```python
from build123d import *

# Parameters (mm, degrees)
SCHIZZO1_R                    = 1.5
SCHIZZO1_W                    = 40
SCHIZZO1_H                    = 10
ESTRUSIONE_ESTRUSIONE1_DEPTH  = 4
RACCORDO1_R                   = 10
SCHIZZO2_R                    = 4
SCHIZZO2_R_2                  = 2
ESTRUSIONE_ESTRUSIONE2_DEPTH  = 4
SCHIZZO3_W                    = 40
SCHIZZO3_H                    = 5
ESTRUSIONE_ESTRUSIONE3_DEPTH  = 20
TAGLIO_ESTRUSIONE1_DEPTH      = 90.673017123
TAGLIO_ESTRUSIONE1_DEPTH_BACK = 90.673017123
SCHIZZO4_R                    = 2.5
SCHIZZO5_W                    = 5
SCHIZZO5_H                    = 60
ESTRUSIONE_ESTRUSIONE4_DEPTH  = 54
SCHIZZO6_R                    = 1.5
ESTRUSIONE_ESTRUSIONE5_DEPTH  = 5
RACCORDO2_R                   = 2
SMUSSO1_SIZE                  = 1
SCHIZZO7_R                    = 1
TAGLIO_ESTRUSIONE2_DEPTH      = 10


with BuildPart() as part:
    # Schizzo1 → Estrusione-Estrusione1 (new body)
    # profile 1 of 5: a face of its own
    with BuildSketch(Plane.XY):
        with BuildLine():
            Line((32.5, -20), (32.5, -10))
            Line((32.5, -10), (32.5, 10))
            Line((32.5, 10), (32.5, 20))
            Line((32.5, 20), (-64, 20))
            ThreePointArc((-64, 20), (-65.5, 18.5), (-67, 20))
            Line((-67, 20), (-72.5, 20))
            Line((-72.5, 20), (-72.5, -20))
            Line((-72.5, -20), (-67, -20))
            ThreePointArc((-67, -20), (-65.5, -18.5), (-64, -20))
            Line((-64, -20), (32.5, -20))
        make_face()
    # profile 2 of 5: a face of its own
    with BuildSketch(Plane.XY):
        with BuildLine():
            Line((-64, 20), (32.5, 20))
            Line((32.5, 20), (32.5, 30))
            Line((32.5, 30), (-72.5, 30))
            Line((-72.5, 30), (-72.5, 20))
            Line((-72.5, 20), (-67, 20))
            ThreePointArc((-67, 20), (-65.5, 21.5), (-64, 20))
        make_face()
        with Locations((4.5, 28)):
            Circle(SCHIZZO1_R, mode=Mode.SUBTRACT)
    # profile 3 of 5: a face of its own
    with BuildSketch(Plane.XY):
        with BuildLine():
            Line((32.5, -30), (32.5, -20))
            Line((32.5, -20), (-64, -20))
            ThreePointArc((-64, -20), (-65.5, -21.5), (-67, -20))
            Line((-67, -20), (-72.5, -20))
            Line((-72.5, -20), (-72.5, -30))
            Line((-72.5, -30), (32.5, -30))
        make_face()
        with Locations((4.5, -28)):
            Circle(SCHIZZO1_R, mode=Mode.SUBTRACT)
    # profile 4 of 5: a face of its own
    with BuildSketch(Plane.XY):
        with Locations((52.5, 15)):
            Rectangle(SCHIZZO1_W, SCHIZZO1_H)
    # profile 5 of 5: a face of its own
    with BuildSketch(Plane.XY):
        with Locations((52.5, -15)):
            Rectangle(SCHIZZO1_W, SCHIZZO1_H)
    extrude(amount=ESTRUSIONE_ESTRUSIONE1_DEPTH)

    # Raccordo1
    raccordo1_edges = [part.edges().sort_by_distance(p)[0] for p in [
        (32.5, 20, 2),
        (32.5, -20, 2),
    ]]
    fillet(raccordo1_edges, radius=RACCORDO1_R - 0.0001)  # a hair under: the kernel refuses the full size

    # Schizzo2 → Estrusione-Estrusione2 (add)
    # profile 1 of 2: a face of its own
    with BuildSketch(Plane.XY.offset(4)):
        with Locations((4.5, -28)):
            Circle(SCHIZZO2_R)
        with Locations((4.5, -28)):
            Circle(SCHIZZO2_R_2, mode=Mode.SUBTRACT)
    # profile 2 of 2: a face of its own
    with BuildSketch(Plane.XY.offset(4)):
        with Locations((4.5, 28)):
            Circle(SCHIZZO2_R)
        with Locations((4.5, 28)):
            Circle(SCHIZZO2_R_2, mode=Mode.SUBTRACT)
    extrude(amount=-ESTRUSIONE_ESTRUSIONE2_DEPTH)

    # Schizzo3 → Estrusione-Estrusione3 (add)
    with BuildSketch(Plane.XY.offset(4)):
        with Locations((52.5, -12.5)):
            Rectangle(SCHIZZO3_W, SCHIZZO3_H)
        with Locations((52.5, 12.5)):
            Rectangle(SCHIZZO3_W, SCHIZZO3_H)
    extrude(amount=ESTRUSIONE_ESTRUSIONE3_DEPTH)

    # Schizzo4 → Taglio-Estrusione1 (cut, two sides: drawn at the far end of the back side and taken through both)
    with BuildSketch(Plane.XZ.offset(15).offset(-TAGLIO_ESTRUSIONE1_DEPTH_BACK)):
        with Locations(Location((42.5, 14, 0), (0, 0, 270))):
            Circle(SCHIZZO4_R)
        with Locations(Location((62.5, 14, 0), (0, 0, 270))):
            Circle(SCHIZZO4_R)
    extrude(amount=TAGLIO_ESTRUSIONE1_DEPTH + TAGLIO_ESTRUSIONE1_DEPTH_BACK, mode=Mode.SUBTRACT)

    # Schizzo5 → Estrusione-Estrusione4 (add)
    with BuildSketch(Plane.XY.offset(4)):
        with Locations((-75, 0)):
            Rectangle(SCHIZZO5_W, SCHIZZO5_H)
    extrude(amount=-ESTRUSIONE_ESTRUSIONE4_DEPTH)

    # Schizzo6 → Estrusione-Estrusione5 (add)
    with BuildSketch(Plane(origin=(0, 0, -50), x_dir=(-1, 0, 0), z_dir=(0, 0, -1))):
        Polygon((87.5, 20), (77.5, 30), (77.5, -30), (87.5, -20), align=None)
        with Locations((82.065858054, -15)):
            Circle(SCHIZZO6_R, mode=Mode.SUBTRACT)
        with Locations((82.065858054, 15)):
            Circle(SCHIZZO6_R, mode=Mode.SUBTRACT)
    extrude(amount=-ESTRUSIONE_ESTRUSIONE5_DEPTH)

    # Raccordo2
    raccordo2_edges = [part.edges().sort_by_distance(p)[0] for p in [
        (32.5, -12.5, 4),
        (52.5, -15, 4),
        (72.5, -12.5, 24),
        (32.5, -12.5, 24),
        (52.5, 15, 4),
        (32.5, 12.5, 4),
        (32.5, 12.5, 24),
        (72.5, 12.5, 24),
        (-77.5, 0, 4),
        (-87.5, 20, -47.5),
        (-87.5, -20, -47.5),
        (-72.5, 0, 0),
        (72.5, 20, 2),
        (72.5, -20, 2),
        (32.5, -30, 2),
        (32.5, 30, 2),
    ]]
    fillet(raccordo2_edges, radius=RACCORDO2_R)

    # Smusso1
    smusso1_edges = [part.edges().sort_by_distance(p)[0] for p in [
        (3, 28, 0),
        (3, -28, 0),
        (-67, 20, 0),
        (-64, -20, 0),
    ]]
    chamfer(smusso1_edges, length=SMUSSO1_SIZE)

    # Schizzo7 → Taglio-Estrusione2 (cut)
    with BuildSketch(Plane.XY.offset(4)):
        with Locations((-75, 0)):
            Circle(SCHIZZO7_R)
        with Locations((-75, 25)):
            Circle(SCHIZZO7_R)
        with Locations((-75, -25)):
            Circle(SCHIZZO7_R)
    extrude(amount=-TAGLIO_ESTRUSIONE2_DEPTH, mode=Mode.SUBTRACT)


solid = part.part
```
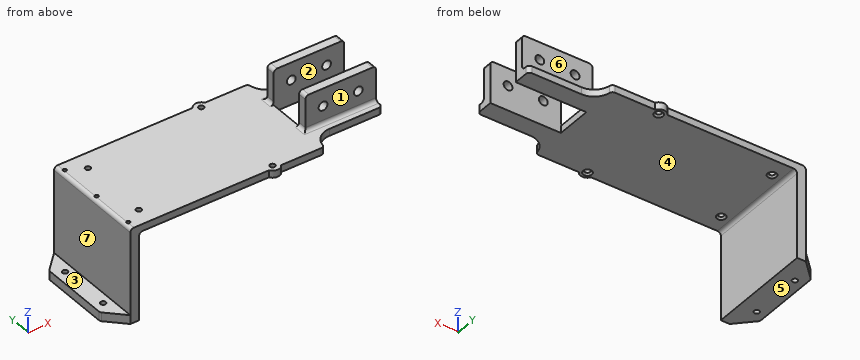
Source: CAD feature listing. Evaluate the final solid. Frame: model axes, mm. Face numbers are marked on the shaded views. A direction names the side the tool comes from. Coordinates: 2 decimals unless noted, no trailing zeros. Loops run counter-clockwise (first coordinate to the right, second up) from the corner with the lowest first, then second, coordinate; pieces in that order, holes last. Notation, with made-up numbers: (-10, 35) - (17, 35) arc R23 ccw to (17, 47) - close; hole circle Ø2 at (69.5, 64.5). An arc over 180 degrees is marked (long way). Answer as CSV lines item,"result".
1. Section C-C (x = -10.5). Return loops of the section in (y, z), then the cut area to 3 significant figures.
Established:
outline,"(-30, 0) - (30, 0) - (30, 4) - (-30, 4) - close"
area,"240 mm2"
2. Ray query, line 1 (X direction, y = -12.45, z = 14); line 2 (Y direction, x = -75, z = -1.25); line 3 (Z direction, x = 42.5, y = 12.5). Return the intervals inside material, ascending.
Established:
line 1,"x = 32.5 to 40, 45 to 60, 65 to 72.5"
line 2,"y = -30 to -26, -24 to -1, 1 to 24, 26 to 30"
line 3,"z = 0 to 11.5, 16.5 to 24"
3. Section B-B (y = -7). Return loops of the section in (x, z), then the cut area to 3 significant figures.
Established:
outline,"(-87.5, -50) - (-72.5, -50) - (-72.5, -2) arc R2 cw to (-70.5, 0) - (32.5, 0) - (32.5, 4) - (-75.5, 4) arc R2 ccw to (-77.5, 2) - (-77.5, -45) - (-87.5, -45) - close"
area,"740 mm2"
4. Mould query, pull axis Y, two halves, no side actions, for the marked faces 1, 2 and 3. Classes: released by +Y, released by -Y, zero draft, split by the parting line, or undercut.
Established:
face 1,"released by -Y"
face 2,"undercut"
face 3,"zero draft"
5. Section D-D (z = -25). Return loops of the section in (x, y), then the cut area to 3 significant figures.
Established:
outline,"(-77.5, -30) - (-72.5, -30) - (-72.5, 30) - (-77.5, 30) - close"
area,"300 mm2"
6. Section A-A (x = 62.5). Return loops of the section in (y, z).
Established:
outline,"(-20, 0) - (-10, 0) - (-10, 11.5) - (-15, 11.5) - (-15, 6) arc R2 cw to (-17, 4) - (-20, 4) - close; (-15, 16.5) - (-10, 16.5) - (-10, 24) - (-15, 24) - close; (10, 0) - (20, 0) - (20, 4) - (17, 4) arc R2 cw to (15, 6) - (15, 11.5) - (10, 11.5) - close; (10, 16.5) - (15, 16.5) - (15, 24) - (10, 24) - close"
7. Contact query for flat-ended pins moving along their axis: pin 1 (3 mm diameter, centred on y = -0.5, z = 2.5, fed in from +X); pin 2 (2.5 mm diameter, centred on x = -82.07, y = -15, fed in from +Z) (3 decimals); pin 3 (1.2 mm diameter, centred on x = 57, z = 1.5, fed in from -Y); pin 4 (6 mm diameter, centred on y = -19, z = -40, fed in from +X). Output: stop coordinate, or through.
Established:
pin 1,"stops at x = 32.5"
pin 2,"passes through"
pin 3,"stops at y = -20"
pin 4,"stops at x = -72.5"
8. Reachability of the marked faces 4, 5, 6 and 7 from +Z, -Z, +X, -X, +Y, -Y: full face, straight path, thin tool, end or side. Return the list, or none.
Established:
face 4,"-Z, +X, +Y, -Y"
face 5,"-Z, +X, -X, +Y, -Y"
face 6,"+Z, +X, -X, +Y"
face 7,"+Z, -X, +Y, -Y"
